The drawing under review shows one solid part. Ordinate dimensions are in mm from its lowest x, y, z. Coordinates: 2 decimals unless noted, no trailing zeros. Loops run counter-clockwise (first coordinate to the right, second up) from the corner with the lowest first, then second, coordinate; pieces in that order, holes last. Notation, with made-up numbers: (-9.75, 38) - (43.25, 38) arc R30 ccw to (43.25, 63) - close; hole circle Ø5 at (39.5, 33.5). An arc over 180 degrees is marked (long way). Answer as a JSON object with one key per item and string values. Group by question number.
Item 1: Mouldability with a two-part tool opening along X and no side actions: class the marked faces 1 and 2 as released by +X, released by -X, zero draft, split by the parting line, or undercut.
Item 2: We need section C-C (z = 9). Give the boundary of the cut face in (x, y).
Item 3: We need section D-D (x = 72). Give the boundary of the cut face in (y, z), then the cut area to 3 significant figures.
Item 4: We need section A-A (y = 7.5). Give the boundary of the cut face in (x, z), then the cut area to 3 significant figures.
Item 5: Clearance check with flat-ended pins moving along their axes: pin 1 (10 mm diameter, centred on x = 64.5, z = 24.5, fed in from +Y); pin 2 (3 mm diameter, centred on y = 7.5, z = 6.5, fed in from -X); pin 3 (1.5 mm diameter, centred on x = 26, y = 9, fed in from +Z). State where each tip first meets the part, or that it passes through.
Item 6: To check wall thickness, follow line 1 (X direction, y = 5.5, z = 8.5); line 2 (X direction, y = 8, z = 11); line 3 (Y direction, x = 87.5, z = 12.5). State the ranges of each line that lie inside material, in increasing order.
Item 7: We need section B-B (x = 50). Give the boundary of the cut face in (y, z).
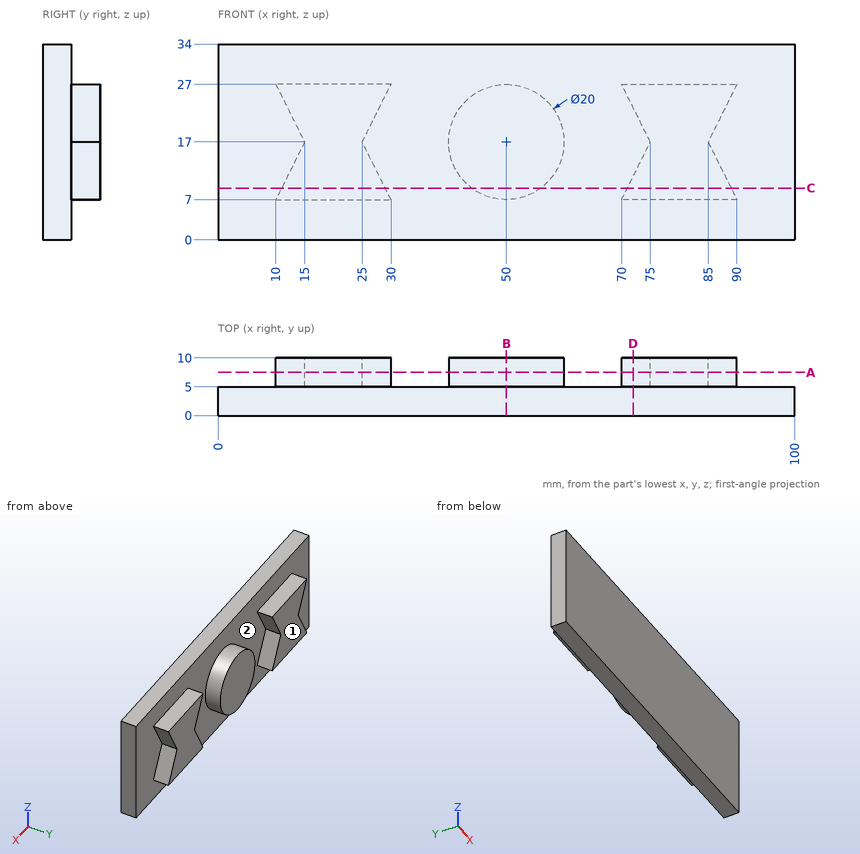
Check sheet entries:
{
 "1": {"face 1": "zero draft", "face 2": "undercut"},
 "2": {"outline": "(0, 0) - (100, 0) - (100, 5) - (89, 5) - (89, 10) - (71, 10) - (71, 5) - (56, 5) - (56, 10) - (44, 10) - (44, 5) - (29, 5) - (29, 10) - (11, 10) - (11, 5) - (0, 5) - close"},
 "3": {"outline": "(0, 0) - (5, 0) - (5, 7) - (10, 7) - (10, 11) - (5, 11) - (5, 23) - (10, 23) - (10, 27) - (5, 27) - (5, 34) - (0, 34) - close", "area": "210 mm2"},
 "4": {"outline": "(10, 7) - (30, 7) - (25, 17) - (30, 27) - (10, 27) - (15, 17) - close; circle Ø20 at (50, 17); (70, 7) - (90, 7) - (85, 17) - (90, 27) - (70, 27) - (75, 17) - close", "area": "914 mm2"},
 "5": {"pin 1": "stops at y = 5", "pin 2": "stops at x = 10", "pin 3": "stops at z = 27"},
 "6": {"line 1": "x = 10.75 to 29.25, 44.73 to 55.27, 70.75 to 89.25", "line 2": "x = 12 to 28, 42 to 58, 72 to 88", "line 3": "y = 0 to 5"},
 "7": {"outline": "(0, 0) - (5, 0) - (5, 7) - (10, 7) - (10, 27) - (5, 27) - (5, 34) - (0, 34) - close"}
}
